from build123d import *

# Parameters (mm, degrees)
SKETCH1_W                 = 155.194
SKETCH1_H                 = 149.606
BOSS_EXTRUDE1_DEPTH       = 2.54
SKETCH2_W                 = 62.103
SKETCH2_H                 = 90.8685
BOSS_EXTRUDE2_DEPTH       = 2.54
SKETCH3_W                 = 2.54
SKETCH3_H                 = 25.4
CUT_EXTRUDE1_DEPTH        = 159.486688428
LPATTERN1_COUNT           = 3
LPATTERN1_PITCH           = 50.8
MIRROR1_COPY_1_SKETCH_W   = 2.54
MIRROR1_COPY_1_SKETCH_H   = 25.4
MIRROR1_COPY_1_DEPTH      = 159.486688428
MIRROR1_COPY_2_SKETCH_W   = 2.54
MIRROR1_COPY_2_SKETCH_H   = 25.4
MIRROR1_COPY_2_DEPTH      = 159.486688428
SKETCH4_W                 = 12.7
SKETCH4_H                 = 2.54
CUT_EXTRUDE2_DEPTH        = 159.486688428
LPATTERN2_COUNT           = 3
LPATTERN2_PITCH           = 25.4
MIRROR2_COPY_1_SKETCH_W   = 12.7
MIRROR2_COPY_1_SKETCH_H   = 2.54
MIRROR2_COPY_1_DEPTH      = 159.486688428
MIRROR2_COPY_2_SKETCH_W   = 12.7
MIRROR2_COPY_2_SKETCH_H   = 2.54
MIRROR2_COPY_2_DEPTH      = 159.486688428
SKETCH5_W                 = 2.54
SKETCH5_H                 = 12.7
CUT_EXTRUDE3_DEPTH        = 2.54
LPATTERN3_COUNT           = 4
LPATTERN3_PITCH           = 25.4
MIRROR3_COPY_1_SKETCH_W   = 2.54
MIRROR3_COPY_1_SKETCH_H   = 12.7
MIRROR3_COPY_1_DEPTH      = 2.54
MIRROR3_COPY_2_SKETCH_W   = 2.54
MIRROR3_COPY_2_SKETCH_H   = 12.7
MIRROR3_COPY_2_DEPTH      = 2.54
MIRROR3_COPY_3_SKETCH_W   = 2.54
MIRROR3_COPY_3_SKETCH_H   = 12.7
MIRROR3_COPY_3_DEPTH      = 2.54
SKETCH6_W                 = 25.019
SKETCH6_H                 = 2.54
CUT_EXTRUDE4_DEPTH        = 2.54
LPATTERN4_COUNT           = 3
LPATTERN4_PITCH           = 50.038
F_6_CLEARANCE_HOLE1_D     = 3.6576
F_6_CLEARANCE_HOLE1_DEPTH = 9.398
F_6_CLEARANCE_HOLE1_TIP   = 1.0988539


with BuildPart() as part:
    # Sketch1 → Boss-Extrude1 (new body)
    with BuildSketch(Plane.XY):
        Rectangle(SKETCH1_W, SKETCH1_H)
    extrude(amount=BOSS_EXTRUDE1_DEPTH)

    # Sketch2 → Boss-Extrude2 (add)
    with BuildSketch(Plane.XY.offset(2.54)):
        with Locations((-108.6485, -29.36875)):
            Rectangle(SKETCH2_W, SKETCH2_H)
    boss_extrude2 = extrude(amount=-BOSS_EXTRUDE2_DEPTH)

    # Sketch3 → Cut-Extrude1 (cut, through all)
    with BuildSketch(Plane.XY.offset(2.54)):
        with Locations((-76.327, 34.163)):
            Rectangle(SKETCH3_W, SKETCH3_H)
    cut_extrude1 = extrude(amount=-CUT_EXTRUDE1_DEPTH, mode=Mode.SUBTRACT)

    # LPattern1: Cut-Extrude1 ×3
    with Locations(*[(0, -i * LPATTERN1_PITCH, 0) for i in range(1, LPATTERN1_COUNT)]):
        add(cut_extrude1, mode=Mode.SUBTRACT)

    # Mirror1: Boss-Extrude2, Cut-Extrude1 across plane
    add(boss_extrude2.mirror(Plane(origin=(0, 0, 0), x_dir=(0, 0, 1), z_dir=(1, 0, 0))))
    add(cut_extrude1.mirror(Plane(origin=(0, 0, 0), x_dir=(0, 0, 1), z_dir=(1, 0, 0))), mode=Mode.SUBTRACT)

    # Mirror1 copy 1 sketch → Mirror1 copy 1 (cut, through all)
    with BuildSketch(Plane(origin=(0, -50.8, 2.54), x_dir=(-1, 0, 0), z_dir=(0, 0, 1))):
        with Locations((-76.327, -34.163)):
            Rectangle(MIRROR1_COPY_1_SKETCH_W, MIRROR1_COPY_1_SKETCH_H)
    extrude(amount=-MIRROR1_COPY_1_DEPTH, mode=Mode.SUBTRACT)

    # Mirror1 copy 2 sketch → Mirror1 copy 2 (cut, through all)
    with BuildSketch(Plane(origin=(0, -101.6, 2.54), x_dir=(-1, 0, 0), z_dir=(0, 0, 1))):
        with Locations((-76.327, -34.163)):
            Rectangle(MIRROR1_COPY_2_SKETCH_W, MIRROR1_COPY_2_SKETCH_H)
    extrude(amount=-MIRROR1_COPY_2_DEPTH, mode=Mode.SUBTRACT)

    # Sketch4 → Cut-Extrude2 (cut, through all)
    with BuildSketch(Plane.XY.offset(2.54)):
        with Locations((-139.7, 14.7955)):
            Rectangle(SKETCH4_W, SKETCH4_H)
    cut_extrude2 = extrude(amount=-CUT_EXTRUDE2_DEPTH, mode=Mode.SUBTRACT)

    # LPattern2: Cut-Extrude2 ×3
    with Locations(*[(i * LPATTERN2_PITCH, 0, 0) for i in range(1, LPATTERN2_COUNT)]):
        add(cut_extrude2, mode=Mode.SUBTRACT)

    # Mirror2: Cut-Extrude2 across plane
    add(cut_extrude2.mirror(Plane(origin=(0, 0, 0), x_dir=(0, 0, 1), z_dir=(1, 0, 0))), mode=Mode.SUBTRACT)

    # Mirror2 copy 1 sketch → Mirror2 copy 1 (cut, through all)
    with BuildSketch(Plane(origin=(-25.4, 0, 2.54), x_dir=(-1, 0, 0), z_dir=(0, 0, 1))):
        with Locations((-139.7, -14.7955)):
            Rectangle(MIRROR2_COPY_1_SKETCH_W, MIRROR2_COPY_1_SKETCH_H)
    extrude(amount=-MIRROR2_COPY_1_DEPTH, mode=Mode.SUBTRACT)

    # Mirror2 copy 2 sketch → Mirror2 copy 2 (cut, through all)
    with BuildSketch(Plane(origin=(-50.8, 0, 2.54), x_dir=(-1, 0, 0), z_dir=(0, 0, 1))):
        with Locations((-139.7, -14.7955)):
            Rectangle(MIRROR2_COPY_2_SKETCH_W, MIRROR2_COPY_2_SKETCH_H)
    extrude(amount=-MIRROR2_COPY_2_DEPTH, mode=Mode.SUBTRACT)

    # Sketch5 → Cut-Extrude3 (cut)
    with BuildSketch(Plane.XY.offset(2.54)):
        with Locations((-138.43, -55.753)):
            Rectangle(SKETCH5_W, SKETCH5_H)
    cut_extrude3 = extrude(amount=-CUT_EXTRUDE3_DEPTH, mode=Mode.SUBTRACT)

    # LPattern3: Cut-Extrude3 ×4
    with Locations(*[(0, i * LPATTERN3_PITCH, 0) for i in range(1, LPATTERN3_COUNT)]):
        add(cut_extrude3, mode=Mode.SUBTRACT)

    # Mirror3: Cut-Extrude3 across plane
    add(cut_extrude3.mirror(Plane(origin=(0, 0, 0), x_dir=(0, 0, 1), z_dir=(1, 0, 0))), mode=Mode.SUBTRACT)

    # Mirror3 copy 1 sketch → Mirror3 copy 1 (cut)
    with BuildSketch(Plane(origin=(0, 25.4, 2.54), x_dir=(-1, 0, 0), z_dir=(0, 0, 1))):
        with Locations((-138.43, 55.753)):
            Rectangle(MIRROR3_COPY_1_SKETCH_W, MIRROR3_COPY_1_SKETCH_H)
    extrude(amount=-MIRROR3_COPY_1_DEPTH, mode=Mode.SUBTRACT)

    # Mirror3 copy 2 sketch → Mirror3 copy 2 (cut)
    with BuildSketch(Plane(origin=(0, 50.8, 2.54), x_dir=(-1, 0, 0), z_dir=(0, 0, 1))):
        with Locations((-138.43, 55.753)):
            Rectangle(MIRROR3_COPY_2_SKETCH_W, MIRROR3_COPY_2_SKETCH_H)
    extrude(amount=-MIRROR3_COPY_2_DEPTH, mode=Mode.SUBTRACT)

    # Mirror3 copy 3 sketch → Mirror3 copy 3 (cut)
    with BuildSketch(Plane(origin=(0, 76.2, 2.54), x_dir=(-1, 0, 0), z_dir=(0, 0, 1))):
        with Locations((-138.43, 55.753)):
            Rectangle(MIRROR3_COPY_3_SKETCH_W, MIRROR3_COPY_3_SKETCH_H)
    extrude(amount=-MIRROR3_COPY_3_DEPTH, mode=Mode.SUBTRACT)

    # Sketch6 → Cut-Extrude4 (cut)
    with BuildSketch(Plane.XY.offset(2.54)):
        with Locations((-50.038, 73.533)):
            Rectangle(SKETCH6_W, SKETCH6_H)
    cut_extrude4 = extrude(amount=-CUT_EXTRUDE4_DEPTH, mode=Mode.SUBTRACT)

    # LPattern4: Cut-Extrude4 ×3
    with Locations(*[(i * LPATTERN4_PITCH, 0, 0) for i in range(1, LPATTERN4_COUNT)]):
        add(cut_extrude4, mode=Mode.SUBTRACT)

    # #6 Clearance Hole1
    with Locations(Plane.XY.offset(2.54)):
        with Locations((-68.072, 62.738), (68.072, 62.738)):
            Hole(F_6_CLEARANCE_HOLE1_D / 2, depth=F_6_CLEARANCE_HOLE1_DEPTH)
            with Locations((0, 0, -(F_6_CLEARANCE_HOLE1_DEPTH + F_6_CLEARANCE_HOLE1_TIP / 2))):  # 118° drill point
                Cone(0, F_6_CLEARANCE_HOLE1_D / 2, F_6_CLEARANCE_HOLE1_TIP, mode=Mode.SUBTRACT)


solid = part.part
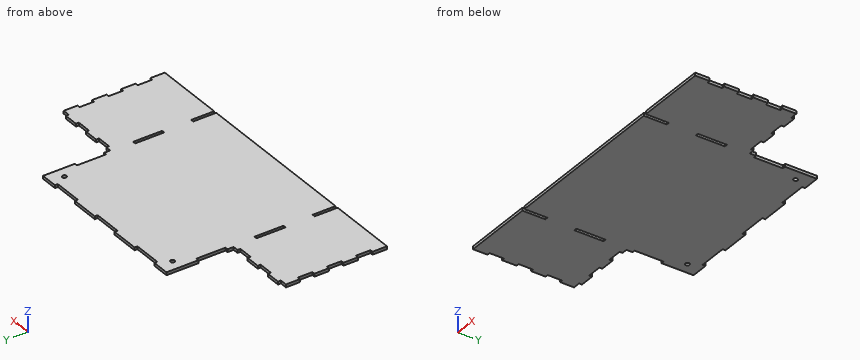
Work out the finished part from the listing and answer in its coordinate system (mm). Round coordinates to 2 decimals unless told otherwise and drop trailing zeros. Write each loop counter-clockwise with the first axis right and the second up, starting at its lowest first coordinate (ties: lowest second). Pieces come first, ordered by that corner, then holes. Notation, with made-up numbers: (78.5, -17) - (101.5, -17) arc R20 ccw to (101.5, 13) - close; hole circle Ø2 at (89, 2.25). An arc over 180 degrees is marked (long way). Answer in a Markdown table with one row per item. Add a question column.
1. A cutting plane is placed at C-C, the plane z = 1.15. Count the separate pieces of the cut face and the enclosed holes in it, and give its area (3 significant figures).
2. A cutting plane is placed at A-A, the plane y = -65. Determine the outline of the cut face in (x, z).
3. Find the intervals of material crossed by line 1 along X through (y, z) = (-8.5, 0.7); line 2 along X through (y, z) = (-23.5, 1.6); line 3 along Y through (x, z) = (-110.5, 1.5), in increasing order. Write a range as from..to.
4. Given pin 1 (1 mm diameter, centred on y = -49.5, z = 0.5, fed in from +X); pin 2 (0.8 mm diameter, centred on x = -1, z = 1.5, fed in from +Y); pin 3 (0.8 mm diameter, centred on x = -104, z = 1, fed in from +Y); pin 4 (0.8 mm diameter, centred on x = -138, z = 0.5, fed in from +Y), each flat-ended and moving along its own axis, determine where each tip first touches the part or whether it passes through.
5. A cutting plane is placed at D-D, the plane y = 32. Determine the outline of the cut face in (x, z), and give its area (3 significant figures).
6. A cutting plane is placed at B-B, the plane x = 87. Determine the outline of the cut face in (y, z).
Worked out:
| question | item | result |
|---|---|---|
| 1 | separate pieces | 1 |
| 1 | enclosed holes | 4 |
| 1 | area | 33,600 mm^2 |
| 2 | outline | (-139.7, 0) - (-77.6, 0) - (-77.6, 2.54) - (-139.7, 2.54) - close; (-75.06, 0) - (75.06, 0) - (75.06, 2.54) - (-75.06, 2.54) - close; (77.6, 0) - (139.7, 0) - (139.7, 2.54) - (77.6, 2.54) - close |
| 3 | line 1 | -137.16..-77.6, -75.06..75.06, 77.6..137.16 |
| 3 | line 2 | -139.7..-77.6, -75.06..75.06, 77.6..139.7 |
| 3 | line 3 | -74.8..13.53 |
| 4 | pin 1 | x = 139.7 |
| 4 | pin 2 | y = 72.26 |
| 4 | pin 3 | y = 16.07 |
| 4 | pin 4 | y = 13.53 |
| 5 | outline | (-75.06, 0) - (75.06, 0) - (75.06, 2.54) - (-75.06, 2.54) - close |
| 5 | area | 381 mm^2 |
| 6 | outline | (-74.8, 0) - (13.53, 0) - (13.53, 2.54) - (-74.8, 2.54) - close |
